Verification items for the finished model (mm, model axes). A direction names the side the tool comes from. Give positions to 0.01 mm unless a question says otherwise; leave off trailing zeros. Loops run counter-clockwise (first coordinate to the right, second up) from the corner with the lowest first, then second, coordinate; pieces in that order, holes last. Notation, with made-up numbers: (54.25, 83) -> (76.25, 83) arc R29 ccw to (76.25, 121) -> close; hole circle Ø11 at (6, 11.25). An arc over 180 degrees is marked (long way). Answer in a Markdown table with one row per item. Add a question column.
Q1. Section check B-B on x = 3.5. Enter the section's corners in (y, z).
Q2. Material ranges on probe 1 along Z at (x, y) = (0, 4.5); probe 2 along Z at (x, y) = (0, 8); probe 3 along Z at (x, y) = (17, 5), recorded low to high.
Q3. Set-up check for faces 4 (the face through (31, 13, 0)), 5 (the face through (-16, 7, 1.5)), 6 (the face through (-22, 6, -7.3)), 7 (the face through (-24.374, 6.084, -9.481)), 8 (the face through (-16, 12, 0)): record each of +Z, -Z, +X, -X, +Y, -Y from which the full face is reachable in a straight line by a thin tool's end or side.
Q4. Gauge pin test, flat ends, axial feed: P1, Ø3, axis at x = 20.5, y = 6, coming from the +Z side; P2, Ø2.5, axis at x = 16, z = 0.5, coming from the +Y side; P3, Ø1.9, axis at y = 8.5, z = 14.5, coming from the -X side. Record the tip position at first contact, or that the pin passes through.
Q5. Release check for a two-part mould opening along X. For faces 1 (the face through (-6.182, 4.684, 23.465)), 2 (the face through (-16, 7, 1.3)), 3 (the face through (31.345, 6.084, -4.873)) record: pulls with the +X half, pulls with the -X half, needs draft (parallel to the pull), parting line crosses it, or undercut.
Q6. Section check A-A on y = 5. Give the number of separate pieces and of enclosed holes in the cut face, and give its area (3 significant figures).
```python
from build123d import *
from build123d.topology import SkipClean

# Parameters (mm, degrees)
SKETCH_1_W          = 42
SKETCH_1_H          = 42
EXTRUDE_1_DEPTH     = 2
EXTRUDE_2_DEPTH     = 0.5
SKETCH_3_R          = 2
SKETCH_3_R_2        = 1
CUT_EXTRUDE_1_DEPTH = 30.803523282
EXTRUDE_START       = -12
EXTRUDE_3_OUTLINE_R = 2
EXTRUDE_3_DEPTH     = 12
EXTRUDE_4_DEPTH     = 2
EXTRUDE_5_DEPTH     = 9.5
DRAFT_1_DEPTH       = 9.5
SKETCH_8_R          = 2
CUT_EXTRUDE_2_DEPTH = 7
CUT_EXTRUDE_3_REACH = 46.272
SKETCH_9_W          = 9.6
SKETCH_9_H          = 14.6
SKETCH_9_W_2        = 9
SKETCH_9_H_2        = 14


# Read off the part's stored shape, not the designer's step: Бобышка-Вытянуть3, Уклон1
with BuildPart() as part:
    # Эскиз1 → Бобышка-Вытянуть1 (new body)
    with BuildSketch(Plane(origin=(0, 0, 0), x_dir=(1, 0, 0), z_dir=(0, 1, 0))):
        Rectangle(SKETCH_1_W, SKETCH_1_H)
    extrude(amount=EXTRUDE_1_DEPTH)

    # Эскиз2 → Бобышка-Вытянуть2 (add)
    with BuildSketch(Plane(origin=(0, 2, 0), x_dir=(1, 0, 0), z_dir=(0, 1, 0))):
        with BuildLine():
            Line((-1.778376117, -14.123475383), (1.778376117, -14.123475383))
            ThreePointArc((1.778376117, -14.123475383), (15.863961031, -15.863961031), (14.123475383, -1.778376117))
            Line((14.123475383, -1.778376117), (14.123475383, 1.778376117))
            ThreePointArc((14.123475383, 1.778376117), (15.863961031, 15.863961031), (1.778376117, 14.123475383))
            Line((1.778376117, 14.123475383), (-1.778376117, 14.123475383))
            ThreePointArc((-1.778376117, 14.123475383), (-15.863961031, 15.863961031), (-14.123475383, 1.778376117))
            Line((-14.123475383, 1.778376117), (-14.123475383, -1.778376117))
            ThreePointArc((-14.123475383, -1.778376117), (-15.863961031, -15.863961031), (-1.778376117, -14.123475383))
        make_face()
    extrude(amount=EXTRUDE_2_DEPTH)

    # Эскиз3 → Вырез-Вытянуть1 (cut, through all)
    # profile 1 of 7: a face of its own
    with BuildSketch(Plane.XZ):
        with Locations(Location((0, -17.5, 0), (0, 0, 270))):
            Circle(SKETCH_3_R)
        with Locations((0, -17.5)):
            Circle(SKETCH_3_R_2, mode=Mode.SUBTRACT)
    # profile 2 of 7: a face of its own
    with BuildSketch(Plane.XZ):
        with BuildLine():
            Line((-21, -21), (-17, -21))
            ThreePointArc((-17, -21), (-19.828427125, -19.828427125), (-21, -17))
            Line((-21, -17), (-21, -21))
        make_face()
    # profile 3 of 7: a face of its own
    with BuildSketch(Plane.XZ):
        with BuildLine():
            ThreePointArc((21, -17), (19.828427125, -19.828427125), (17, -21))
            Line((17, -21), (21, -21))
            Line((21, -21), (21, -17))
        make_face()
    # profile 4 of 7: a face of its own
    with BuildSketch(Plane.XZ):
        with BuildLine():
            Line((21, 21), (19, 21))
            ThreePointArc((19, 21), (20.414213562, 20.414213562), (21, 19))
            Line((21, 19), (21, 21))
        make_face()
    # profile 5 of 7: a face of its own
    with BuildSketch(Plane.XZ):
        with Locations(Location((0, 17.5, 0), (0, 0, 270))):
            Circle(SKETCH_3_R)
        with Locations((0, 17.5)):
            Circle(SKETCH_3_R_2, mode=Mode.SUBTRACT)
    # profile 6 of 7: a face of its own
    with BuildSketch(Plane.XZ):
        with Locations((0, 17.5)):
            Circle(SKETCH_3_R_2)
    # profile 7 of 7: a face of its own
    with BuildSketch(Plane.XZ):
        with BuildLine():
            Line((-21, 21), (-21, 19))
            ThreePointArc((-21, 19), (-20.414213562, 20.414213562), (-19, 21))
            Line((-19, 21), (-21, 21))
        make_face()
    extrude(amount=-CUT_EXTRUDE_1_DEPTH, mode=Mode.SUBTRACT)


with BuildPart() as cut_extrude_1_kept_piece:
    # of the separate pieces the step leaves, the one the design keeps (cut_extrude_1_pieces_kept)
    add(part.part.solids().sort_by_distance((-19, 0, 21))[0])

    # Бобышка-Вытянуть3 outline → Бобышка-Вытянуть3 (add)
    with SkipClean():  # the faces are left unmerged after this step: merging them gives an invalid solid
        with BuildSketch(Plane.XZ.offset(EXTRUDE_START)):
            with BuildLine():
                Line((-22, -12.611663805), (-21, -12.611663805))
                Line((-21, -12.611663805), (-21, -17))
                ThreePointArc((-21, -17), (-19.828427125, -19.828427125), (-17, -21))
                Line((-17, -21), (17, -21))
                ThreePointArc((17, -21), (19.828427125, -19.828427125), (21, -17))
                Line((21, -17), (21, -12.611663805))
                Line((21, -12.611663805), (22, -12.611663805))
                ThreePointArc((22, -12.611663805), (24.332770191, -9.517506551), (27.666666667, -7.542472333))
                ThreePointArc((27.666666667, -7.542472333), (31.384371141, -4.820768106), (32.984359711, -0.5))
                Line((32.984359711, -0.5), (32.984359711, 0.5))
                ThreePointArc((32.984359711, 0.5), (31.384371141, 4.820768106), (27.666666667, 7.542472333))
                ThreePointArc((27.666666667, 7.542472333), (24.332770191, 9.517506551), (22, 12.611663805))
                Line((22, 12.611663805), (21, 12.611663805))
                Line((21, 12.611663805), (21, 19))
                ThreePointArc((21, 19), (20.414213562, 20.414213562), (19, 21))
                Line((19, 21), (-19, 21))
                ThreePointArc((-19, 21), (-20.414213562, 20.414213562), (-21, 19))
                Line((-21, 19), (-21, 12.611663805))
                Line((-21, 12.611663805), (-22, 12.611663805))
                ThreePointArc((-22, 12.611663805), (-24.332770191, 9.517506551), (-27.666666667, 7.542472333))
                ThreePointArc((-27.666666667, 7.542472333), (-31.384371141, 4.820768106), (-32.984359711, 0.5))
                Line((-32.984359711, 0.5), (-32.984359711, -0.5))
                ThreePointArc((-32.984359711, -0.5), (-31.384371141, -4.820768106), (-27.666666667, -7.542472333))
                ThreePointArc((-27.666666667, -7.542472333), (-24.332770191, -9.517506551), (-22, -12.611663805))
            make_face()
            with BuildLine():
                Line((-26.8, 7.3), (-21, 7.3))
                Line((-21, 7.3), (-21, 5.123475383))
                ThreePointArc((-21, 5.123475383), (-23.765130637, 6.381621867), (-26.8, 6.245798588))
                Line((-26.8, 6.245798588), (-26.8, 7.3))
            make_face(mode=Mode.SUBTRACT)
            with BuildLine():
                Line((14.623475383, -1.5), (14.623475383, 1.5))
                Line((14.623475383, 1.5), (18.67544468, 1.5))
                ThreePointArc((18.67544468, 1.5), (18.652597901, 1.400173775), (18.631326669, 1.3))
                Line((18.631326669, 1.3), (14.823475383, 1.3))
                Line((14.823475383, 1.3), (14.823475383, -1.3))
                Line((14.823475383, -1.3), (18.631326669, -1.3))
                ThreePointArc((18.631326669, -1.3), (18.652597901, -1.400173775), (18.67544468, -1.5))
                Line((18.67544468, -1.5), (14.623475383, -1.5))
            make_face(mode=Mode.SUBTRACT)
            with Locations((0, 17.5)):
                Circle(EXTRUDE_3_OUTLINE_R, mode=Mode.SUBTRACT)
            with Locations((0, -17.5)):
                Circle(EXTRUDE_3_OUTLINE_R, mode=Mode.SUBTRACT)
            with BuildLine():
                Line((-14.623475383, -1.5), (-18.67544468, -1.5))
                ThreePointArc((-18.67544468, -1.5), (-18.652597901, -1.400173775), (-18.631326669, -1.3))
                Line((-18.631326669, -1.3), (-14.823475383, -1.3))
                Line((-14.823475383, -1.3), (-14.823475383, 1.3))
                Line((-14.823475383, 1.3), (-18.631326669, 1.3))
                ThreePointArc((-18.631326669, 1.3), (-18.652597901, 1.400173775), (-18.67544468, 1.5))
                Line((-18.67544468, 1.5), (-14.623475383, 1.5))
                Line((-14.623475383, 1.5), (-14.623475383, -1.5))
            make_face(mode=Mode.SUBTRACT)
        extrude(amount=EXTRUDE_3_DEPTH)

    # Эскиз6 → Бобышка-Вытянуть4 (add)
    with SkipClean():  # the faces are left unmerged after this step: merging them gives an invalid solid
        with BuildSketch(Plane(origin=(0, 12, 0), x_dir=(1, 0, 0), z_dir=(0, 1, 0))):
            with BuildLine():
                ThreePointArc((-19.161948935, -1.384615385), (-19, 0), (-19.161948935, 1.384615385))
                ThreePointArc((-19.161948935, 1.384615385), (-19.949874575, 3.239789066), (-21.307692308, 4.729361892))
                ThreePointArc((-21.307692308, 4.729361892), (-31, 0), (-21.307692308, -4.729361892))
                ThreePointArc((-21.307692308, -4.729361892), (-19.949874575, -3.239789066), (-19.161948935, -1.384615385))
            make_face()
            with BuildLine():
                ThreePointArc((19.161948935, 1.384615385), (19, 0), (19.161948935, -1.384615385))
                ThreePointArc((19.161948935, -1.384615385), (19.949874575, -3.239789066), (21.307692308, -4.729361892))
                ThreePointArc((21.307692308, -4.729361892), (31, 0), (21.307692308, 4.729361892))
                ThreePointArc((21.307692308, 4.729361892), (19.949874575, 3.239789066), (19.161948935, 1.384615385))
            make_face()
        extrude(amount=EXTRUDE_4_DEPTH)

    # Эскиз7 → Бобышка-Вытянуть5 (add)
    with SkipClean():  # the faces are left unmerged after this step: merging them gives an invalid solid
        with BuildSketch(Plane.XZ):
            with BuildLine():
                Line((0, 22), (0, 21))
                Line((0, 21), (5, 21))
                Line((5, 21), (5, 26))
                Line((5, 26), (0, 26))
                Line((0, 26), (0, 25))
                ThreePointArc((0, 25), (1.060660172, 24.560660172), (1.5, 23.5))
                ThreePointArc((1.5, 23.5), (1.060660172, 22.439339828), (0, 22))
            make_face()
            with BuildLine():
                Line((-5, 21), (0, 21))
                Line((0, 21), (0, 22))
                ThreePointArc((0, 22), (-1.5, 23.5), (0, 25))
                Line((0, 25), (0, 26))
                Line((0, 26), (-5, 26))
                Line((-5, 26), (-5, 21))
            make_face()
        extrude(amount=-EXTRUDE_5_DEPTH)

    # Уклон1 outline → Уклон1 (add)
    with SkipClean():  # the faces are left unmerged after this step: merging them gives an invalid solid
        with BuildSketch(Plane(origin=(0, 0, 0), x_dir=(1, 0, 0), z_dir=(0, 1, 0))):
            Polygon((-5, -21), (-7.331538291, -21), (-5, -26), align=None)
            Polygon((7.331538291, -21), (5, -21), (5, -26), align=None)
        extrude(amount=DRAFT_1_DEPTH)

    # Эскиз8 → Вырез-Вытянуть2 (cut)
    with SkipClean():  # the faces are left unmerged after this step: merging them gives an invalid solid
        with BuildSketch(Plane.XZ):
            with Locations(Location((0, 23.5, 0), (0, 0, 270))):
                Circle(SKETCH_8_R)
        extrude(amount=-CUT_EXTRUDE_2_DEPTH, mode=Mode.SUBTRACT)

    # Эскиз9 → Вырез-Вытянуть3 (cut, up to next)
    with BuildSketch(Plane.XZ, mode=Mode.PRIVATE) as cut_extrude_3_sk1:
        with Locations((-22, 0)):
            Rectangle(SKETCH_9_W, SKETCH_9_H)
        with Locations((-22, 0)):
            Rectangle(SKETCH_9_W_2, SKETCH_9_H_2, mode=Mode.SUBTRACT)
    cut_extrude_3_tool1 = extrude(cut_extrude_3_sk1.sketch, amount=-CUT_EXTRUDE_3_REACH, mode=Mode.PRIVATE) & cut_extrude_1_kept_piece.part
    # Эскиз9 → Вырез-Вытянуть3 (cut, up to next)
    with BuildSketch(Plane.XZ, mode=Mode.PRIVATE) as cut_extrude_3_sk2:
        with Locations((-22, 0)):
            Rectangle(SKETCH_9_W_2, SKETCH_9_H_2)
    cut_extrude_3_tool2 = extrude(cut_extrude_3_sk2.sketch, amount=-CUT_EXTRUDE_3_REACH, mode=Mode.PRIVATE) & cut_extrude_1_kept_piece.part
    # Эскиз9 → Вырез-Вытянуть3 (cut, up to next)
    with BuildSketch(Plane.XZ, mode=Mode.PRIVATE) as cut_extrude_3_sk3:
        with Locations((22, 0)):
            Rectangle(SKETCH_9_W, SKETCH_9_H)
        with Locations((22, 0)):
            Rectangle(SKETCH_9_W_2, SKETCH_9_H_2, mode=Mode.SUBTRACT)
    cut_extrude_3_tool3 = extrude(cut_extrude_3_sk3.sketch, amount=-CUT_EXTRUDE_3_REACH, mode=Mode.PRIVATE) & cut_extrude_1_kept_piece.part
    # Эскиз9 → Вырез-Вытянуть3 (cut, up to next)
    with BuildSketch(Plane.XZ, mode=Mode.PRIVATE) as cut_extrude_3_sk4:
        with Locations((22, 0)):
            Rectangle(SKETCH_9_W_2, SKETCH_9_H_2)
    cut_extrude_3_tool4 = extrude(cut_extrude_3_sk4.sketch, amount=-CUT_EXTRUDE_3_REACH, mode=Mode.PRIVATE) & cut_extrude_1_kept_piece.part
    add(cut_extrude_3_tool1.solids().sort_by_distance((-26.625266, 0, 0))[0], mode=Mode.SUBTRACT)
    add(cut_extrude_3_tool2.solids().sort_by_distance((-22, 0, 0))[0], mode=Mode.SUBTRACT)
    add(cut_extrude_3_tool3.solids().sort_by_distance((17.374734, 0, 0))[0], mode=Mode.SUBTRACT)
    add(cut_extrude_3_tool4.solids().sort_by_distance((22, 0, 0))[0], mode=Mode.SUBTRACT)


solid = cut_extrude_1_kept_piece.part
```
Taken from the geometry:
| question | item | result |
|---|---|---|
| 1 | outline | (0, -21) -> (12, -21) -> (12, 21) -> (9.5, 21) -> (9.5, 26) -> (0, 26) -> close |
| 2 | probe 1 | z = -21 to -19.5, -15.5 to 15.5, 19.5 to 21.5, 25.5 to 26 |
| 2 | probe 2 | z = -21 to -19.5, -15.5 to 15.5, 19.5 to 22, 25 to 26 |
| 2 | probe 3 | z = -21 to -1.5, -1.3 to 1.3, 1.5 to 21 |
| 3 | face 4 | +X, +Y |
| 3 | face 5 | +Y |
| 3 | face 6 | +Y, -Y |
| 3 | face 7 | -Z, -X, +Y, -Y |
| 3 | face 8 | +Z, -Z, +Y |
| 4 | P1 | stops at z = 21 |
| 4 | P2 | stops at y = 12 |
| 4 | P3 | stops at x = -21 |
| 5 | face 1 | pulls with the -X half |
| 5 | face 2 | undercut |
| 5 | face 3 | pulls with the +X half |
| 6 | separate pieces | 3 |
| 6 | enclosed holes | 5 |
| 6 | area | 1,880 mm² |
